Autodesk Inventor part; units mm, degrees
ref_plane "YZ Plane" through (0, 0, 0) normal (1, 0, 0) x (0, 1, 0)
ref_plane "XZ Plane" through (0, 0, 0) normal (0, 1, 0) x (-1, 0, 0)
ref_plane "XY Plane" through (0, 0, 0) normal (0, 0, 1) x (1, 0, 0)
sketch "Szkic1" plane through (0, 0, 0) normal (0, 0, 1) x (1, 0, 0)
  circle A0 centre (0, 0) radius 5
  line L0 (-21.5, 5) -> (-21.5, -5)
  line L1 (21.5, 5) -> (21.5, -5)
  circle A1 centre (0, 0) radius 10
  line L2 (-21.5, -5) -> (-2.3932, -9.7094)
  line L3 (21.5, -5) -> (2.3932, -9.7094)
  line L4 (-7.5, 13.5) -> (7.5, 13.5)
  line L5 (-21.5, 5) -> (-7.5, 8.4507)
  line L6 (21.5, 5) -> (7.5, 8.4507)
  line L7 (-7.5, 13.5) -> (-7.5, 6.6144)
  line L8 (7.5, 13.5) -> (7.5, 6.6144)
  dimension "d0" = 10
  dimension "d1" = 43
  dimension "d2" = 10
  dimension "d3" = 10
  dimension "d4" = 5
  dimension "d5" = 21.5
  dimension "d6" = 20
  dimension "d7" = 13.5
  dimension "d8" = 7.5
  dimension "d9" = 15
extrude "Wyciągnięcie proste1" add sketch "Szkic1" along normal blind 5 contours L5 L7 A1 L2 L0 | A1 L8 L6 L1 L3
extrude "Wyciągnięcie proste2" add sketch "Szkic1" along normal blind 10 contours L7 L4 L8 A1 | A1
fillet "Zaokrąglenie1" radius 8 2 edges at (7.5, 6.6144, 7.5) (-7.5, 6.6144, 7.5)
fillet "Zaokrąglenie2" radius 2 4 edges at (21.5, 5, 2.5) (21.5, -5, 2.5) (-21.5, -5, 2.5) (-21.5, 5, 2.5)
sketch "Szkic2" plane through (0, 0, 10) normal (0, 0, 1) x (1, 0, 0)
  line L0 (-0.5, 2.515) -> (0.5, 2.515)
  line L1 (0.5, 2.515) -> (0.5, 16.0792)
  line L2 (0.5, 16.0792) -> (-0.5, 16.0792)
  line L3 (-0.5, 16.0792) -> (-0.5, 2.515)
  point P0 (0, 0)
  dimension "d16" = 1
  dimension "d17" = 0.5
extrude "Wyciągnięcie proste3" cut sketch "Szkic2" against normal through all
fillet "Zaokrąglenie3" radius 0.6 4 edges at (-7.5, 13.5, 5) (-0.5, 13.5, 5) (0.5, 13.5, 5) (7.5, 13.5, 5)
sketch "Szkic3" plane through (0, 0, 5) normal (0, 0, 1) x (1, 0, 0)
  arc A0 (-19.9786, 5.375) -> (-21.5, 3.4331) centre (-19.5, 3.4331) ccw
  line L0 (-21.5, 3.4331) -> (-21.5, -3.4331)
  arc A1 (-21.5, -3.4331) -> (-19.9786, -5.375) centre (-19.5, -3.4331) ccw
  line L1 (-19.9786, -5.375) -> (-2.3932, -9.7094)
  arc A2 (-8.6111, 5.0842) -> (-2.3932, -9.7094) centre (0, 0) ccw
  arc A3 (-8.6111, 5.0842) -> (-7.5314, 8.4429) centre (-15.5, 9.1515) ccw
  line L2 (-7.5314, 8.4429) -> (-19.9786, 5.375)
  arc A4 (19.9786, -5.375) -> (21.5, -3.4331) centre (19.5, -3.4331) ccw
  line L3 (21.5, -3.4331) -> (21.5, 3.4331)
  arc A5 (21.5, 3.4331) -> (19.9786, 5.375) centre (19.5, 3.4331) ccw
  line L4 (19.9786, 5.375) -> (7.5314, 8.4429)
  arc A6 (7.5314, 8.4429) -> (8.6111, 5.0842) centre (15.5, 9.1515) ccw
  arc A7 (2.3932, -9.7094) -> (8.6111, 5.0842) centre (0, 0) ccw
  line L5 (2.3932, -9.7094) -> (19.9786, -5.375)
  point P0 (-16, 0)
  point P1 (16, 0)
  dimension "d21" = 32
  dimension "d22" = 43
  dimension "d23" = 5.5
hole "Otwór1" at (-16, 0, 5) at (16, 0, 5) direction (0, 0, -1) diameter 5 end through all
chamfer "Faza1" distance 1 angle 45 2 edges at (-16, 2.5, 5) (16, 2.5, 5)
equation "\"d3\" = d2"
properties part number "COTS_GENERIC_SHF10_Linear_Rail_Mount"
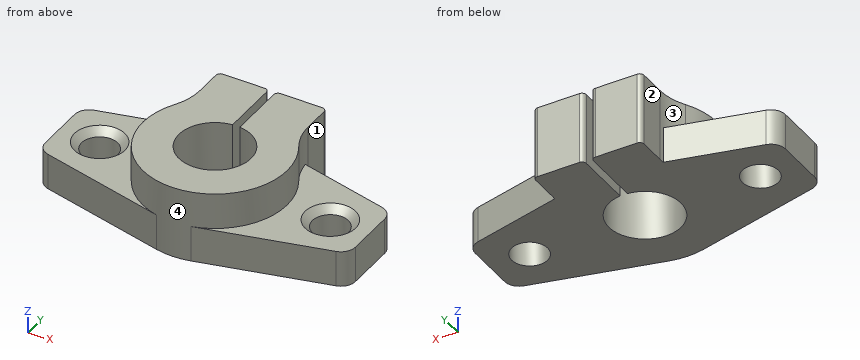
Geometry: final body of the model. Coordinates: model frame, mm. Face numbers are marked on the shaded views. A direction names the side the tool comes from. Give positions to 0.01 mm unless a question says otherwise; leave off trailing zeros. Write each loop counter-clockwise with the first axis right and the second up, starting at its lowest first coordinate (ties: lowest second). Pieces come first, ordered by that corner, then holes. Notation, with made-up numbers: (-38.5, 53) -> (-5.5, 53) arc R25 cw to (-5.5, 91) -> close; hole circle Ø1 at (-35.75, 84). An arc over 180 degrees is marked (long way). Answer in a Markdown table with one row per item.
(1) Set-up query: the marked faces 1, 2, 3 and 4. Return all of +Z, -Z, +X, -X, +Y, -Y with unobstructed straight access to the full face (end or side cutting, diameter ignored); none if empty.
Answers below:
| item | result |
|---|---|
| face 1 | +Z, -Z, +X, +Y |
| face 2 | +Z, -Z, -X, +Y |
| face 3 | +Z, -X, +Y |
| face 4 | +Z |
(2) Ray query, line 1 along X through (y, z) = (0, 2.2); line 2 along X through (y, z) = (12.75, 5); line 3 along X through (y, z) = (0, 5.75). Return the intervals inside material, ascending. Write a range as [from, to].
Answers below:
| item | result |
|---|---|
| line 1 | [-21.5, -18.5], [-13.5, -5], [5, 13.5], [18.5, 21.5] |
| line 2 | [-7.5, -0.5], [0.5, 7.5] |
| line 3 | [-10, -5], [5, 10] |
(3) Section query C-C on x = -16. Return loops of the section in (y, z), then the cut area to 3 significant figures.
Answers below:
| item | result |
|---|---|
| outline | (-6.36, 0) -> (-2.5, 0) -> (-2.5, 4) -> (-3.5, 5) -> (-6.36, 5) -> close; (2.5, 0) -> (6.36, 0) -> (6.36, 5) -> (3.5, 5) -> (2.5, 4) -> close |
| area | 37.6 mm^2 |
(4) Section query D-D on y = 0. Return loops of the section in (x, z), then the cut area to 3 significant figures.
Answers below:
| item | result |
|---|---|
| outline | (-21.5, 0) -> (-18.5, 0) -> (-18.5, 4) -> (-19.5, 5) -> (-21.5, 5) -> close; (-13.5, 0) -> (-5, 0) -> (-5, 10) -> (-10, 10) -> (-10, 5) -> (-12.5, 5) -> (-13.5, 4) -> close; (5, 0) -> (13.5, 0) -> (13.5, 4) -> (12.5, 5) -> (10, 5) -> (10, 10) -> (5, 10) -> close; (18.5, 0) -> (21.5, 0) -> (21.5, 5) -> (19.5, 5) -> (18.5, 4) -> close |
| area | 163 mm^2 |
(5) Section query A-A on y = 10. Return loops of the section in (x, z).
Answers below:
| item | result |
|---|---|
| outline | (-7.5, 0) -> (-0.5, 0) -> (-0.5, 10) -> (-7.5, 10) -> close; (0.5, 0) -> (7.5, 0) -> (7.5, 10) -> (0.5, 10) -> close |
(6) Pin query (flat end, axial travel): pin 1 (6 mm diameter, centred on y = -2, z = 7, fed in from +X); pin 2 (8 mm diameter, centred on x = 16, y = 0, fed in from +Z); pin 3 (3 mm diameter, centred on x = 2, z = 8.5, fed in from -Y); pin 4 (5 mm diameter, centred on x = -4.5, z = 1.5, fed in from -Y). Return the tip coordinate at first contact, or that it passes through.
Answers below:
| item | result |
|---|---|
| pin 1 | x = 21.5 |
| pin 2 | z = 5 |
| pin 3 | y = -9.99 |
| pin 4 | y = -9.8 |
(7) Section query B-B on z = 1.5. Return loops of the section in (x, y).
Answers below:
| item | result |
|---|---|
| outline | (-21.5, -3.43) arc R2 ccw to (-19.98, -5.37) -> (-2.39, -9.71) arc R10 ccw to (2.39, -9.71) -> (19.98, -5.37) arc R2 ccw to (21.5, -3.43) -> (21.5, 3.43) arc R2 ccw to (19.98, 5.37) -> (7.53, 8.44) arc R8 cw to (7.5, 9.15) -> (7.5, 12.9) arc R0.6 ccw to (6.9, 13.5) -> (1.1, 13.5) arc R0.6 ccw to (0.5, 12.9) -> (0.5, 4.97) arc R5 cw (long way) to (-0.5, 4.97) -> (-0.5, 12.9) arc R0.6 ccw to (-1.1, 13.5) -> (-6.9, 13.5) arc R0.6 ccw to (-7.5, 12.9) -> (-7.5, 9.15) arc R8 cw to (-7.53, 8.44) -> (-19.98, 5.37) arc R2 ccw to (-21.5, 3.43) -> close; hole circle Ø5 at (-16, 0); hole circle Ø5 at (16, 0) |
